from build123d import *

# Parameters (mm, degrees)
SKETCH2_W           = 100
SKETCH2_H           = 48
SKETCH2_R           = 2
BOSS_EXTRUDE1_DEPTH = 65


with BuildPart() as part:
    # Sketch2 → Boss-Extrude1 (new body)
    with BuildSketch(Plane(origin=(0, 0, 0), x_dir=(1, 0, 0), z_dir=(0, 1, 0))):
        Rectangle(SKETCH2_W, SKETCH2_H)
        with Locations(Location((-29, 0, 0), (0, 0, 270))):
            Circle(SKETCH2_R, mode=Mode.SUBTRACT)
        with Locations(Location((0, 0, 0), (0, 0, 270))):
            Circle(SKETCH2_R, mode=Mode.SUBTRACT)
        with Locations(Location((29, 0, 0), (0, 0, 270))):
            Circle(SKETCH2_R, mode=Mode.SUBTRACT)
    extrude(amount=-BOSS_EXTRUDE1_DEPTH)


solid = part.part
The listing builds one solid part. Answer for the finished solid, in the listing's coordinates (mm). Coordinates: 2 decimals unless noted, no trailing zeros. Order: outer loops, then holes, each group sorted by start corner. A loop starts at its lowest first (then second) coordinate and runs counter-clockwise, first axis right, second up.
Q1. A cutting plane is placed at A-A, the plane x = 0. Write down the section's boundary in (y, z), and give its area (3 significant figures).
Q2. For a pull along X with two mould halves and no side action, classify faces 1 (the face through (-31, -32, 0)), 2 (the face through (50, -32, 0)), 3 (the face through (-50, -32, 0)), 4 (the face through (-1, -32, 24)) as pulls with the +X half, pulls with the -X half, needs draft (parallel to the pull), parting line crosses it, or undercut.
Q3. Consider line 1 (X direction, y = -40, z = 0); line 2 (Z direction, x = 1, y = -35.5); line 3 (Z direction, x = 1.5, y = -12.5). Determine where each line is inside the solid, lowest interval first.
Q4. A cutting plane is placed at B-B, the plane z = 0. Write down the section's boundary in (x, y).
Answers follow:
1. outline: (-65, -24) - (0, -24) - (0, -2) - (-65, -2) - close; (-65, 2) - (0, 2) - (0, 24) - (-65, 24) - close
1. area: 2,860 mm2
2. face 1: undercut
2. face 2: pulls with the +X half
2. face 3: pulls with the -X half
2. face 4: needs draft
3. line 1: x = -50 to -31, -27 to -2, 2 to 27, 31 to 50
3. line 2: z = -24 to -1.73, 1.73 to 24
3. line 3: z = -24 to -1.32, 1.32 to 24
4. outline: (-50, -65) - (-31, -65) - (-31, 0) - (-50, 0) - close; (-27, -65) - (-2, -65) - (-2, 0) - (-27, 0) - close; (2, -65) - (27, -65) - (27, 0) - (2, 0) - close; (31, -65) - (50, -65) - (50, 0) - (31, 0) - close
